from build123d import *

# Parameters (mm, degrees)
SKETCH_1_W      = 33
SKETCH_1_H      = 21
SKETCH_1_W_2    = 29
SKETCH_1_H_2    = 17
EXTRUDE_1_DEPTH = 2
SKETCH_2_W      = 2
SKETCH_2_H      = 2
EXTRUDE_2_DEPTH = 20
SKETCH_3_W      = 33
SKETCH_3_H      = 21
SKETCH_3_W_2    = 29
SKETCH_3_H_2    = 2
SKETCH_3_H_3    = 3
EXTRUDE_6_DEPTH = 2
FILLET_2_R      = 1


with BuildPart() as part:
    # 草图1 → 凸台-拉伸1 (new body)
    with BuildSketch(Plane(origin=(0, 0, 0), x_dir=(1, 0, 0), z_dir=(0, 1, 0))):
        with Locations((16.5, -10.5)):
            Rectangle(SKETCH_1_W, SKETCH_1_H)
        with Locations((16.5, -10.5)):
            Rectangle(SKETCH_1_W_2, SKETCH_1_H_2, mode=Mode.SUBTRACT)
    extrude(amount=EXTRUDE_1_DEPTH)

    # 草图2 → 凸台-拉伸2 (add)
    with BuildSketch(Plane(origin=(0, 2, 0), x_dir=(1, 0, 0), z_dir=(0, 1, 0))):
        with Locations((1, -15)):
            Rectangle(SKETCH_2_W, SKETCH_2_H)
        with Locations((1, -20)):
            Rectangle(SKETCH_2_W, SKETCH_2_H)
        with Locations((1, -1)):
            Rectangle(SKETCH_2_W, SKETCH_2_H)
        with Locations((32, -1)):
            Rectangle(SKETCH_2_W, SKETCH_2_H)
        with Locations((32, -20)):
            Rectangle(SKETCH_2_W, SKETCH_2_H)
        with Locations((32, -15)):
            Rectangle(SKETCH_2_W, SKETCH_2_H)
        with Locations((1, -10)):
            Rectangle(SKETCH_2_W, SKETCH_2_H)
        with Locations((32, -10)):
            Rectangle(SKETCH_2_W, SKETCH_2_H)
        with Locations((1, -5)):
            Rectangle(SKETCH_2_W, SKETCH_2_H)
        with Locations((32, -5)):
            Rectangle(SKETCH_2_W, SKETCH_2_H)
        with Locations((5.5, -1)):
            Rectangle(SKETCH_2_W, SKETCH_2_H)
        with Locations((10, -1)):
            Rectangle(SKETCH_2_W, SKETCH_2_H)
        with Locations((14.5, -1)):
            Rectangle(SKETCH_2_W, SKETCH_2_H)
        with Locations((19, -1)):
            Rectangle(SKETCH_2_W, SKETCH_2_H)
        with Locations((23.5, -1)):
            Rectangle(SKETCH_2_W, SKETCH_2_H)
        with Locations((28, -1)):
            Rectangle(SKETCH_2_W, SKETCH_2_H)
    extrude(amount=EXTRUDE_2_DEPTH)

    # 草图3 → 凸台-拉伸6 (add)
    with BuildSketch(Plane(origin=(0, 22, 0), x_dir=(1, 0, 0), z_dir=(0, 1, 0))):
        with Locations((16.5, -10.5)):
            Rectangle(SKETCH_3_W, SKETCH_3_H)
        with Locations((16.5, -3)):
            Rectangle(SKETCH_3_W_2, SKETCH_3_H_2, mode=Mode.SUBTRACT)
        with Locations((16.5, -7.5)):
            Rectangle(SKETCH_3_W_2, SKETCH_3_H_3, mode=Mode.SUBTRACT)
        with Locations((16.5, -12.5)):
            Rectangle(SKETCH_3_W_2, SKETCH_3_H_3, mode=Mode.SUBTRACT)
        with Locations((16.5, -17.5)):
            Rectangle(SKETCH_3_W_2, SKETCH_3_H_3, mode=Mode.SUBTRACT)
    extrude(amount=EXTRUDE_6_DEPTH)

    # 圆角2
    fillet_2_edges = [part.edges().sort_by_distance(p)[0] for p in [
        (33, 12, 11),
        (33, 12, 9),
        (0, 12, 4),
        (0, 12, 6),
        (33, 12, 6),
        (33, 12, 4),
        (6.5, 12, 0),
        (4.5, 12, 0),
        (11, 12, 0),
        (9, 12, 0),
        (15.5, 12, 0),
        (13.5, 12, 0),
        (20, 12, 0),
        (18, 12, 0),
        (24.5, 12, 0),
        (22.5, 12, 0),
        (29, 12, 0),
        (27, 12, 0),
        (33, 24, 10.5),
        (16.5, 24, 0),
        (16.5, 24, 21),
        (0, 24, 10.5),
        (0, 12, 19),
        (0, 12, 2),
        (2, 12, 0),
        (33, 12, 2),
        (31, 12, 0),
        (33, 12, 19),
        (0, 12, 14),
        (0, 12, 16),
        (0, 12, 0),
        (33, 12, 0),
        (33, 12, 21),
        (0, 12, 21),
        (33, 12, 16),
        (33, 12, 14),
        (0, 12, 9),
        (0, 12, 11),
    ]]
    fillet(fillet_2_edges, radius=FILLET_2_R - 0.0001)  # a hair under: the kernel refuses the full size


solid = part.part
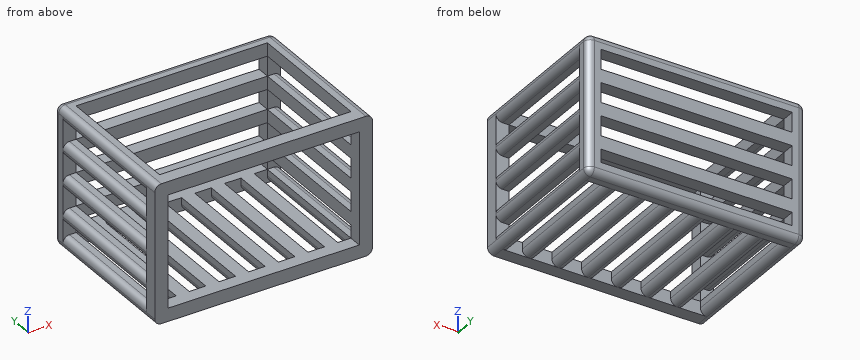
Build history of the part. All positions in model axes, mm. Round coordinates to 2 decimals unless told otherwise and drop trailing zeros. Loops run counter-clockwise (first coordinate to the right, second up) from the corner with the lowest first, then second, coordinate; pieces in that order, holes last. Notation, with made-up numbers: (16.5, -38) -> (46.5, -38) arc R23 ccw to (46.5, -2) -> close; hole circle Ø5 at (78, 0). An arc over 180 degrees is marked (long way). One line per item, written item: value. Start each with the question number.
Q1. Cut at B-B on z = 17. List the corners of the cut face in (x, y).
Q2. Cut at A-A on x = 26.5. Count the separate pieces of the cut face and the enclosed holes in it, plus the area to 3 significant figures.
Q3. Drop flat-ended pins along their axis: pin 1 Ø5 at (x, y) = (19, 6) entering from +Z; pin 2 Ø0.8 at (y, z) = (15.5, 1.5) entering from -X (3 decimals). Give the stop position or say it passes through.
Q4. Probe line 1 along Z through (x, y) = (26, 22.25); line 2 along Y through (x, z) = (21, 20); line 3 along X through (y, z) = (12.25, 10). List the from-to ranges inside material, lowest first.
Q5. Cut at C-C on y = 1.5. List the corners of the cut face in (x, z).
Computed:
1. outline: (0, 0) -> (2, 0) -> (2, 2) -> (0, 2) -> close; (0, 22) -> (2, 22) -> (2, 24) -> (1, 24) arc R1 ccw to (0, 23) -> close; (31, 0) -> (33, 0) -> (33, 2) -> (31, 2) -> close; (31, 22) -> (33, 22) -> (33, 23) arc R1 ccw to (32, 24) -> (31, 24) -> close
2. separate pieces: 7
2. enclosed holes: 0
2. area: 27.6 mm²
3. pin 1: z = 2
3. pin 2: x = 0.005
4. line 1: 0 to 2, 4 to 6, 9 to 11, 14 to 16, 19 to 21
4. line 2: 0 to 2, 22 to 24
4. line 3: 0 to 2, 31 to 33
5. outline: (0, 1) arc R1 ccw to (1, 0) -> (32, 0) arc R1 ccw to (33, 1) -> (33, 20) arc R1 ccw to (32, 21) -> (1, 21) arc R1 ccw to (0, 20) -> close; hole (2, 2) -> (31, 2) -> (31, 19) -> (2, 19) -> close
